from build123d import *

# Parameters (mm, degrees)
EXTRUDE_1_DEPTH     = 42
SKETCH_2_R          = 11
CUT_EXTRUDE_1_DEPTH = 76.286120899
SKETCH_3_R          = 1.5
CUT_EXTRUDE_2_DEPTH = 77.367532368
SKETCH_4_R          = 1.5
CUT_EXTRUDE_3_DEPTH = 76.126559884


with BuildPart() as part:
    # 草图1 → 凸台-拉伸1 (new body)
    with BuildSketch(Plane(origin=(0, 0, 0), x_dir=(0, 0, -1), z_dir=(1, 0, 0))):
        Polygon((0, 2), (0, 0), (2, 0), (42, 0), (42, 2), (2, 2), (2, 48), (0, 48), align=None)
    extrude(amount=EXTRUDE_1_DEPTH)

    # 草图2 → 切除-拉伸1 (cut, through all)
    with BuildSketch(Plane(origin=(0, 0, -2), x_dir=(-1, 0, 0), z_dir=(0, 0, -1))):
        with Locations(Location((-21, 27, 0), (0, 0, 90))):
            Circle(SKETCH_2_R)
    extrude(amount=-CUT_EXTRUDE_1_DEPTH, mode=Mode.SUBTRACT)

    # 草图3 → 切除-拉伸2 (cut, through all)
    with BuildSketch(Plane.XY):
        with Locations((21, 41)):
            Circle(SKETCH_3_R)
        with Locations((21, 13)):
            Circle(SKETCH_3_R)
        with Locations((35, 27)):
            Circle(SKETCH_3_R)
        with Locations((7, 27)):
            Circle(SKETCH_3_R)
    extrude(amount=-CUT_EXTRUDE_2_DEPTH, mode=Mode.SUBTRACT)

    # 草图4 → 切除-拉伸3 (cut, through all)
    with BuildSketch(Plane(origin=(0, 2, 0), x_dir=(1, 0, 0), z_dir=(0, 1, 0))):
        with Locations(Location((5.5, 37, 0), (0, 0, 270))):
            Circle(SKETCH_4_R)
        with Locations(Location((36.5, 37, 0), (0, 0, 270))):
            Circle(SKETCH_4_R)
        with Locations(Location((36.5, 6, 0), (0, 0, 270))):
            Circle(SKETCH_4_R)
        with Locations(Location((5.5, 6, 0), (0, 0, 270))):
            Circle(SKETCH_4_R)
    extrude(amount=-CUT_EXTRUDE_3_DEPTH, mode=Mode.SUBTRACT)


solid = part.part
Can you work these out from the model? Positions are in its coordinate system, mm. A direction names the side the tool comes from. Give positions to 0.01 mm unless a question says otherwise; leave off trailing zeros. Loops run counter-clockwise (first coordinate to the right, second up) from the corner with the lowest first, then second, coordinate; pieces in that order, holes last. Notation, with made-up numbers: M 35.25,-2 L 78.25,-2 A11 cw 78.25,13 Z; hole C 80.5,27.25 d3. An arc over 180 degrees is marked long. One line per item, written item: value. Start each with the question number.
1) If we section it at B-B, the plane z = -37: Write out the boundary of the cut face in (x, y), and give its area (3 significant figures).
2) Thinking about a two-plate mould opening in Z: for faces 1 (the face through (21, 1, -42)), 2 (the face through (42, 13, -1)), 3 (the face through (35.6, 1, -38.2)), 4 (the face through (35, 1, -6)), which applies, +Z half, -Z half, draft (parallel to the pull), parting line (faces both ways), or undercut?
3) On a 3-axis mill with a long thin cutter (end or side, diameter ignored), from which of +Z, -Z, +X, -X, +Y, -Y can I reach the whole of each face in a straight line? I mean faces 5 (the face through (21, 2, -22)), 6 (the face through (21, 0, -21)). Say none if no direction works.
4) If we section it at D-D, the plane x = 39.5: Write out the boundary of the cut face in (y, z).
5) I'm going to push flat-ended pins straight in: pin 1 (4 mm diameter, centred on x = 35, y = 27, fed in from -Z); pin 2 (8 mm diameter, centred on x = 23, y = 9, fed in from +Z); pin 3 (4 mm diameter, centred on x = 36.5, z = -37, fed in from +Y). Where does each tip first touch, or does it pass through?
6) If we section it at A-A, the plane y = 41: Write out the boundary of the cut face in (x, z).
7) If we section it at C-C, the plane x = 21: Write out the boundary of the cut face in (y, z).
8) If I drill on line 1 (X direction, y = 1.45, z = -6); line 2 (Y direction, x = 35, z = -0.55); line 3 (Y direction, x = 7, z = -6.5), over which ranges is the centre line in solid material (lowest first)? Write a range as [from, to].
Completed:
1. outline: M 0,0 L 4,0 L 4,2 L 0,2 Z; M 7,0 L 35,0 L 35,2 L 7,2 Z; M 38,0 L 42,0 L 42,2 L 38,2 Z
1. area: 72.0 mm^2
2. face 1: -Z half
2. face 2: draft
2. face 3: undercut
2. face 4: undercut
3. face 5: -Z, +X, -X, +Y
3. face 6: +Z, -Z, +X, -X, -Y
4. outline: M 0,-42 L 2,-42 L 2,-2 L 48,-2 L 48,0 L 0,0 Z
5. pin 1: stops at z = -2
5. pin 2: stops at z = 0
5. pin 3: stops at y = 2
6. outline: M 0,-2 L 19.5,-2 L 19.5,0 L 0,0 Z; M 22.5,-2 L 42,-2 L 42,0 L 22.5,0 Z
7. outline: M 0,-42 L 2,-42 L 2,-2 L 11.5,-2 L 11.5,0 L 0,0 Z; M 14.5,-2 L 16,-2 L 16,0 L 14.5,0 Z; M 38,-2 L 39.5,-2 L 39.5,0 L 38,0 Z; M 42.5,-2 L 48,-2 L 48,0 L 42.5,0 Z
8. line 1: x = [0, 4], [7, 35], [38, 42]
8. line 2: y = [0, 25.5], [28.5, 48]
8. line 3: y = [0, 2]
